Job drawing, mm, ordinate dimensions from the low corner. One solid piece. A direction names the side the tool comes from. Coordinates: 2 decimals unless noted, no trailing zeros. Order: outer loops, then holes, each group sorted by start corner. A loop starts at its lowest first (then second) coordinate and runs counter-clockwise, first axis right, second up. Notation, with made-up numbers: (42.5, 30.25) - (80.5, 30.25) arc R27 ccw to (80.5, 48.25) - close; hole circle Ø8 at (76.25, 35.25). An arc over 180 degrees is marked (long way). Return JSON: item names as keys, results as strings.
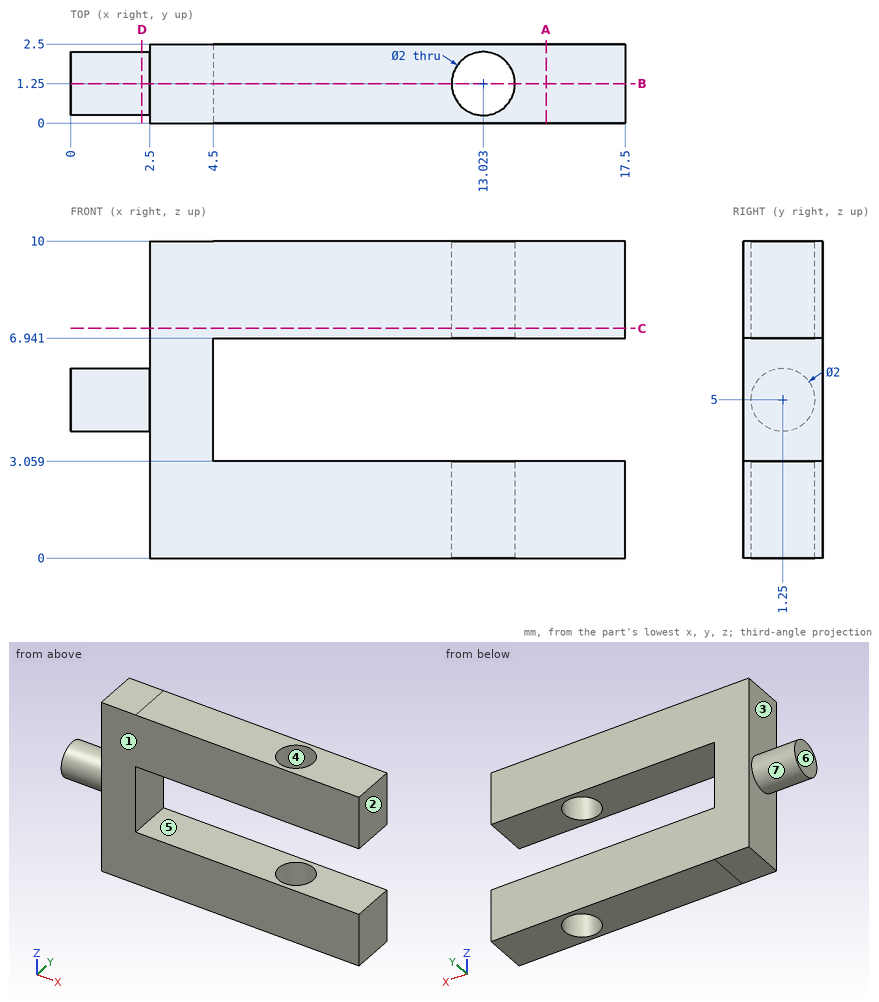
1. Cut at D-D on x = 2.25. Give the cut face in (y, z).
Check values:
{"outline": "circle Ø2 at (1.25, 5)"}
2. Cut at C-C on z = 7.25. Give the cut face in (x, y).
Check values:
{"outline": "(2.5, 0) - (17.5, 0) - (17.5, 2.5) - (2.5, 2.5) - close; hole circle Ø2 at (13.02, 1.25)"}
3. Tool access for the marked faces 5, 6 and 7: list every direction of +Z, -Z, +X, -X, +Y, -Y with a clear straight run to the whole face (end or side of a thin tool).
Check values:
{"face 5": "+X, +Y, -Y", "face 6": "+Z, -Z, -X, +Y, -Y", "face 7": "-X"}
4. Drop flat-ended pins along their axis: pin 1 (1.5 mm diameter, centred on x = 5.5, z = 5, fed in from -Y); pin 2 (0.8 mm diameter, centred on y = 0.5, z = 5.5, fed in from +X). Give the stop position or say it passes through.
Check values:
{"pin 1": "through", "pin 2": "x = 4.5"}
5. Cut at A-A on x = 15. Give the cut face in (y, z), plus the area to 3 significant figures.
Check values:
{"outline": "(0, 0) - (2.5, 0) - (2.5, 3.06) - (0, 3.06) - close; (0, 6.94) - (2.5, 6.94) - (2.5, 10) - (0, 10) - close", "area": "15.3 mm²"}
6. Cut at B-B on y = 1.25. Give the cut face in (x, z).
Check values:
{"outline": "(0, 4) - (2.5, 4) - (2.5, 0) - (12.02, 0) - (12.02, 3.06) - (4.5, 3.06) - (4.5, 6.94) - (12.02, 6.94) - (12.02, 10) - (2.5, 10) - (2.5, 6) - (0, 6) - close; (14.02, 0) - (17.5, 0) - (17.5, 3.06) - (14.02, 3.06) - close; (14.02, 6.94) - (17.5, 6.94) - (17.5, 10) - (14.02, 10) - close"}
7. Probe L1, parallel to Z at x = 14.5, y = 1.55; L2, parallel to X at y = 1.6, z = 8; L3, parallel to X at y = 1.65, z = 8.5. List the from-to ranges inside material, lowest first.
Check values:
{"L1": "0 to 3.06, 6.94 to 10", "L2": "2.5 to 12.09, 13.96 to 17.5", "L3": "2.5 to 12.11, 13.94 to 17.5"}
8. Mould opens along X. For the marked faces 1, 2, 3 and 4 say: pulls with the +X half, pulls with the -X half, needs draft (parallel to the pull), parting line crosses it, or undercut.
Check values:
{"face 1": "needs draft", "face 2": "pulls with the +X half", "face 3": "pulls with the -X half", "face 4": "undercut"}
